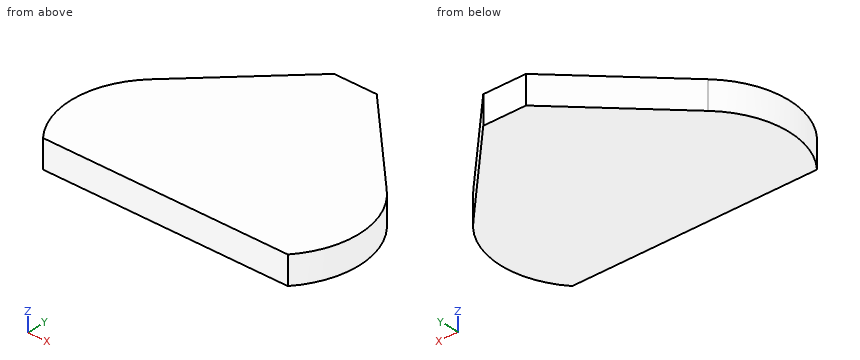
```python
from build123d import *

# Parameters (mm, degrees)
EXTRUSION008_DEPTH = 15
RECTANGLE001_W     = 146.971653
RECTANGLE001_H     = 26.042151
EXTRUSION007_DEPTH = 15
CIRCLE002_R        = 46
EXTRUSION005_DEPTH = 15
CIRCLE003_R        = 46
EXTRUSION006_DEPTH = 15


with BuildPart() as extrusion008:
    # Wire001 → Extrusion008 (new body)
    with BuildSketch(Plane(origin=(-40.513268, 32.899851, 15), x_dir=(1, 0, 0), z_dir=(0, 0, 1))):
        Polygon((0, 0), (51.871842, 51.871844), (74.871842, 51.871844), (126.743685, 1e-06), align=None)
    extrude(amount=-EXTRUSION008_DEPTH)


with BuildPart() as extrusion007:
    # Rectangle001 → Extrusion007 (new body)
    with BuildSketch(Plane(origin=(-43.712536, -55.376318, 15), x_dir=(1, 0, 0), z_dir=(0, 0, 1))):
        with Locations((73.485827, 13.021076)):
            Rectangle(RECTANGLE001_W, RECTANGLE001_H)
    extrude(amount=-EXTRUSION007_DEPTH)


with BuildPart() as extrusion005:
    # Circle002 → Extrusion005 (new body)
    with BuildSketch(Plane(origin=(53.57846, 0.542169, 15), x_dir=(1, 0, 0), z_dir=(0, 0, 1))):
        Circle(CIRCLE002_R)
    extrude(amount=-EXTRUSION005_DEPTH)


with BuildPart() as fusion001002003:
    # Circle003 → Extrusion006 (new body)
    with BuildSketch(Plane(origin=(-8.183821, 0.175382, 15), x_dir=(1, 0, 0), z_dir=(0, 0, 1))):
        Circle(CIRCLE003_R)
    extrude(amount=-EXTRUSION006_DEPTH)

    # Fusion001002002: union Extrusion005
    add(extrusion005.part)

    # Cut: cut Extrusion007
    add(extrusion007.part, mode=Mode.SUBTRACT)

    # Fusion001002003: union Extrusion008
    add(extrusion008.part)


solid = fusion001002003.part
```
Geometry check sheet. Reference: the model listing, model coordinates, mm. Coordinates: 2 decimals unless noted, no trailing zeros. Write each loop counter-clockwise with the first axis right and the second up, starting at its lowest first coordinate (ties: lowest second). Pieces come first, ordered by that corner, then holes. Notation, with made-up numbers: M -17.75,32 L 7.25,32 A23 ccw 7.25,54 Z; hole C -23,33.25 d8. An arc over 180 degrees is marked long. One line per item, written item: value. Start each with the question number.
(1) Scan lines: line 1 along X through (y, z) = (-1, 2.75); line 2 along Y through (x, z) = (8, 11.75); line 3 along Y through (x, z) = (91.5, 8). Record each from-to range of solid material in increasing order. Write a range as [from, to].
(2) Sectioned sample at B-B, the plane y = 26. Enter the section's corners in (x, z).
(3) Sectioned sample at C-C, the plane x = -32. Enter the section's corners in (y, z).
(4) Depth check by flat-ended pin: pin 1 (6 mm diameter, centred on y = 1, z = 7, fed in from -X); pin 2 (5 mm diameter, centred on x = 67, z = 10, fed in from +Y); pin 3 (1.5 mm diameter, centred on y = 45.5, z = 5.5, fed in from +X). Enter the tip coordinate at first touch or a pass-through.
Filled sheet:
1. line 1: [-54.17, 99.55]
1. line 2: [-29.33, 81.41]
1. line 3: [-25.5, 26.58]
2. outline: M -46.25,0 L 91.89,0 L 91.89,15 L -46.25,15 Z
3. outline: M -29.33,0 L 41.41,0 L 41.41,15 L -29.33,15 Z
4. pin 1: x = -54.18
4. pin 2: y = 54.63
4. pin 3: x = 74.38
